For this review, take the finished solid that the model builds, in its own axes (mm). Face numbers are marked on the shaded views. A direction names the side the tool comes from. Coordinates: 2 decimals unless noted, no trailing zeros. Loops run counter-clockwise (first coordinate to the right, second up) from the corner with the lowest first, then second, coordinate; pieces in that order, holes last. Notation, with made-up numbers: (41.5, -28) - (53.5, -28) arc R15 ccw to (53.5, -21) - close; hole circle Ø7 at (39.25, -31.75). An arc over 180 degrees is marked (long way). Answer as a JSON object with one key per item and string values. Group by question number.
Item 1: We need section B-B (x = -9). State how many separate pieces and enclosed holes the cut face has, then the cut area to 3 significant figures.
Item 2: To check wall thickness, follow line 1 (Y direction, x = -11, z = 9.65); line 2 (Z direction, x = 3.25, y = 6.5); line 3 (Z direction, x = -8.5, y = -7.5). State the ranges of each line that lie inside material, in increasing order.
Item 3: Mouldability with a two-part tool opening along X and no side actions: class the marked faces 5, 6 and 7 as released by +X, released by -X, zero draft, split by the parting line, or undercut.
Item 4: We need section A-A (z = 3.5). Give the boundary of the cut face in (x, y), then the cut area to 3 significant figures.
Item 5: Tool access review of the marked faces 1, 2, 3 and 4: name each direction out of +Z, -Z, +X, -X, +Y, -Y from which nothing blocks a thin tool from reaching the whole face with its end or side.
Item 6: Clearance check with flat-ended pins moving along their axes: pin 1 (2.5 mm diameter, centred on x = -8, y = -8, fed in from +Z); pin 2 (6 mm diameter, centred on y = 3.5, z = 3.5, fed in from +X); pin 3 (10.5 mm diameter, centred on x = 0, y = 0, fed in from -Z); pin 4 (1.2 mm diameter, centred on x = 5.5, z = 9.5, fed in from +Y). State where each tip first meets the part, or that it passes through.
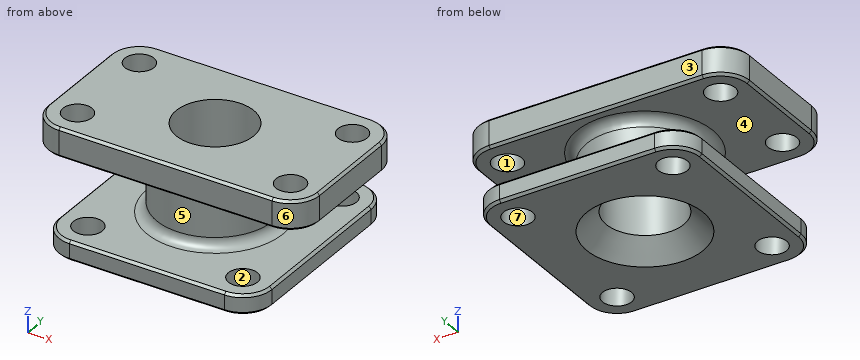
from build123d import *

# Parameters (mm, degrees)
SKETCH1_R           = 1.5
BOSS_EXTRUDE1_DEPTH = 2
SKETCH2_R           = 6
BOSS_EXTRUDE2_DEPTH = 6
SKETCH3_R           = 1.5
BOSS_EXTRUDE3_DEPTH = 3
SKETCH4_R           = 4
CUT_EXTRUDE1_DEPTH  = 21.928449536
CHAMFER1_SIZE       = 2
FILLET1_R           = 1
CHAMFER2_SIZE       = 0.25


with BuildPart() as part:
    # Sketch1 → Boss-Extrude1 (new body)
    with BuildSketch(Plane.XY):
        with BuildLine():
            Line((8, -11), (-8, -11))
            ThreePointArc((-8, -11), (-10.121320344, -10.121320344), (-11, -8))
            Line((-11, -8), (-11, 8))
            ThreePointArc((-11, 8), (-10.121320344, 10.121320344), (-8, 11))
            Line((-8, 11), (8, 11))
            ThreePointArc((8, 11), (10.121320344, 10.121320344), (11, 8))
            Line((11, 8), (11, -8))
            ThreePointArc((11, -8), (10.121320344, -10.121320344), (8, -11))
        make_face()
        with Locations((-8, 8)):
            Circle(SKETCH1_R, mode=Mode.SUBTRACT)
        with Locations((8, 8)):
            Circle(SKETCH1_R, mode=Mode.SUBTRACT)
        with Locations((8, -8)):
            Circle(SKETCH1_R, mode=Mode.SUBTRACT)
        with Locations((-8, -8)):
            Circle(SKETCH1_R, mode=Mode.SUBTRACT)
    extrude(amount=BOSS_EXTRUDE1_DEPTH)

    # Sketch2 → Boss-Extrude2 (add)
    with BuildSketch(Plane.XY.offset(2)):
        Circle(SKETCH2_R)
    extrude(amount=BOSS_EXTRUDE2_DEPTH)

    # Sketch3 → Boss-Extrude3 (add)
    with BuildSketch(Plane.XY.offset(8)):
        with BuildLine():
            Line((11, -8), (-11, -8))
            ThreePointArc((-11, -8), (-13.121320344, -7.121320344), (-14, -5))
            Line((-14, -5), (-14, 5))
            ThreePointArc((-14, 5), (-13.121320344, 7.121320344), (-11, 8))
            Line((-11, 8), (11, 8))
            ThreePointArc((11, 8), (13.121320344, 7.121320344), (14, 5))
            Line((14, 5), (14, -5))
            ThreePointArc((14, -5), (13.121320344, -7.121320344), (11, -8))
        make_face()
        with Locations((-11, 5)):
            Circle(SKETCH3_R, mode=Mode.SUBTRACT)
        with Locations((11, 5)):
            Circle(SKETCH3_R, mode=Mode.SUBTRACT)
        with Locations((11, -5)):
            Circle(SKETCH3_R, mode=Mode.SUBTRACT)
        with Locations((-11, -5)):
            Circle(SKETCH3_R, mode=Mode.SUBTRACT)
    extrude(amount=BOSS_EXTRUDE3_DEPTH)

    # Sketch4 → Cut-Extrude1 (cut, through all)
    with BuildSketch(Plane(origin=(0, 0, 0), x_dir=(-1, 0, 0), z_dir=(0, 0, -1))):
        Circle(SKETCH4_R)
    extrude(amount=-CUT_EXTRUDE1_DEPTH, mode=Mode.SUBTRACT)

    # Chamfer1
    chamfer1_edges = [part.edges().sort_by_distance(p)[0] for p in [
        (4, 0, 0),
    ]]
    chamfer(chamfer1_edges, length=CHAMFER1_SIZE)

    # Fillet1
    fillet1_edges = [part.edges().sort_by_distance(p)[0] for p in [
        (-6, 0, 2),
        (-6, 0, 8),
    ]]
    fillet(fillet1_edges, radius=FILLET1_R)

    # Chamfer2
    chamfer2_edges = [part.edges().sort_by_distance(p)[0] for p in [
        (-11, 0, 0),
        (-10.121320344, 10.121320344, 0),
        (0, 11, 0),
        (10.121320344, 10.121320344, 0),
        (-10.121320344, 10.121320344, 2),
        (-11, 0, 2),
        (-10.121320344, -10.121320344, 2),
        (0, -11, 2),
        (10.121320344, -10.121320344, 2),
        (11, 0, 2),
        (-13.121320344, -7.121320344, 11),
        (0, -8, 11),
        (13.121320344, -7.121320344, 11),
        (14, 0, 11),
        (13.121320344, 7.121320344, 11),
        (0, 8, 11),
        (-13.121320344, 7.121320344, 11),
        (-14, 0, 11),
        (10.121320344, 10.121320344, 2),
        (-13.121320344, -7.121320344, 8),
        (0, -8, 8),
        (13.121320344, -7.121320344, 8),
        (14, 0, 8),
        (13.121320344, 7.121320344, 8),
        (0, 8, 8),
        (-13.121320344, 7.121320344, 8),
        (-14, 0, 8),
        (11, 0, 0),
        (0, 11, 2),
        (10.121320344, -10.121320344, 0),
        (0, -11, 0),
        (-10.121320344, -10.121320344, 0),
    ]]
    chamfer(chamfer2_edges, length=CHAMFER2_SIZE)


solid = part.part
Check sheet entries:
{
 "1": {"separate pieces": "4", "enclosed holes": "0", "area": "82.1 mm2"},
 "2": {"line 1": "y = -8 to -6.5, -3.5 to 3.5, 6.5 to 8", "line 2": "z = 0 to 2, 8 to 11", "line 3": "z = 8 to 11"},
 "3": {"face 5": "split by the parting line", "face 6": "released by +X", "face 7": "undercut"},
 "4": {"outline": "circle Ø12 at (0, 0); hole circle Ø8 at (0, 0)", "area": "62.8 mm2"},
 "5": {"face 1": "+Z", "face 2": "-Z", "face 3": "+Z, +X, -X, +Y", "face 4": "none"},
 "6": {"pin 1": "stops at z = 11", "pin 2": "stops at x = 11", "pin 3": "stops at z = 0.75", "pin 4": "stops at y = 8"}
}
